For this review, take the finished solid that the model builds, in its own axes (mm). Face numbers are marked on the shaded views. A direction names the side the tool comes from. Give positions to 0.01 mm unless a question says otherwise; leave off trailing zeros. Write each loop counter-clockwise with the first axis right and the second up, starting at its lowest first coordinate (ties: lowest second). Pieces come first, ordered by that corner, then holes. Notation, with made-up numbers: M 73.5,54.5 L 95.5,54.5 A26 cw 95.5,86.5 Z; hole C 79.25,40 d2. An arc over 180 degrees is marked long. One line per item, written item: value. Start each with the question number.
Item 1: Consider section D-D, the plane z = 32.1. Write out the cut boundary in (x, y).
Item 2: Consider section C-C, the plane z = 14.9. Write out the cut boundary in (x, y), and give its area (3 significant figures).
Item 3: Consider section A-A, the plane x = -19.3. Write out the cut boundary in (y, z), and give its area (3 significant figures).
Item 4: Clearance check with flat-ended pins moving along their axes: pin 1 Ø16 at (x, z) = (-3.5, 25) entering from -Y; pin 2 Ø16 at (x, z) = (-7, 0.5) entering from -Y. State where each tip first meets the part, or that it passes through.
Item 5: Consider section B-B, the plane x = 0. Write out the cut boundary in (y, z).
Item 6: To check wall thickness, follow probe 1 along Z at (x, y) = (-34.4, -1.1); probe 2 along Z at (x, y) = (-20, -2.55); probe 3 along Z at (x, y) = (7.5, -4.6). State the ranges of each line that lie inside material, in increasing order.
Item 7: Tool access review of the marked faces 4 and 5: name each direction out of +Z, -Z, +X, -X, +Y, -Y from which nothing blocks a thin tool from reaching the whole face with its end or side.
Item 8: Mouldability with a two-part tool opening along X and no side actions: class the marked faces 1, 2 and 3 as released by +X, released by -X, zero draft, split by the parting line, or undercut.
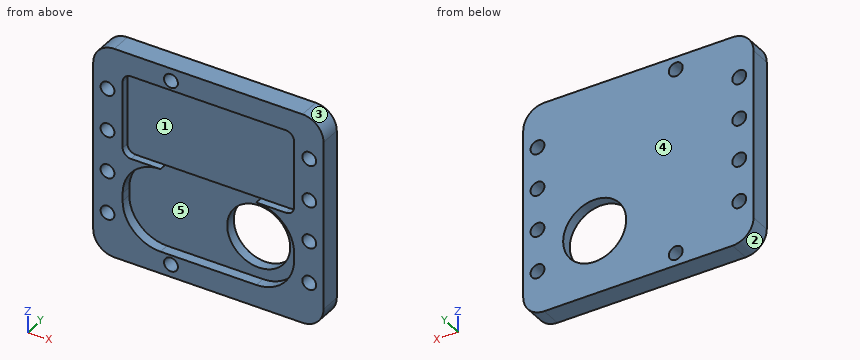
```python
from build123d import *

# Parameters (mm, degrees)
EXTRUSION1_DEPTH        = 5
ENL_V_MAT_EXTRU_2_DEPTH = 2.5
ENL_V_MAT_EXTRU_4_DEPTH = 1.8
ESQUISSE7_R             = 7.5
ENL_V_MAT_EXTRU_3_DEPTH = 52.643973511
TROU_TARAUD_M4X0_71_D   = 3.3


with BuildPart() as part:
    # Esquisse1 → Extrusion1 (new body)
    with BuildSketch(Plane(origin=(0, 0, 0), x_dir=(1, 0, 0), z_dir=(0, 1, 0))):
        with BuildLine():
            Line((-32.8, -35.1), (12, -35.1))
            ThreePointArc((12, -35.1), (15.535533906, -33.635533906), (17, -30.1))
            Line((17, -30.1), (17, 10.2))
            ThreePointArc((17, 10.2), (15.535533906, 13.735533906), (12, 15.2))
            Line((12, 15.2), (-32.8, 15.2))
            ThreePointArc((-32.8, 15.2), (-36.335533906, 13.735533906), (-37.8, 10.2))
            Line((-37.8, 10.2), (-37.8, -30.1))
            ThreePointArc((-37.8, -30.1), (-36.335533906, -33.635533906), (-32.8, -35.1))
        make_face()
    extrude(amount=-EXTRUSION1_DEPTH)

    # Esquisse6 → Enlèv. mat.-Extru.2 (cut)
    with BuildSketch(Plane.XZ.offset(5)):
        with BuildLine():
            Line((1, 9.95), (-21.8, 9.95))
            ThreePointArc((-21.8, 9.95), (-28.163961031, 7.313961031), (-30.8, 0.95))
            Line((-30.8, 0.95), (-30.8, -0.95))
            ThreePointArc((-30.8, -0.95), (-28.163961031, -7.313961031), (-21.8, -9.95))
            Line((-21.8, -9.95), (1, -9.95))
            ThreePointArc((1, -9.95), (7.363961031, -7.313961031), (10, -0.95))
            Line((10, -0.95), (10, 0.95))
            ThreePointArc((10, 0.95), (7.363961031, 7.313961031), (1, 9.95))
        make_face()
    extrude(amount=-ENL_V_MAT_EXTRU_2_DEPTH, mode=Mode.SUBTRACT)

    # Esquisse10 → Enlèv. mat.-Extru.4 (cut)
    with BuildSketch(Plane.XZ.offset(5)):
        with BuildLine():
            Line((8, 9.95), (-28.8, 9.95))
            ThreePointArc((-28.8, 9.95), (-30.214213562, 10.535786438), (-30.8, 11.95))
            Line((-30.8, 11.95), (-30.8, 27.85))
            ThreePointArc((-30.8, 27.85), (-30.214213562, 29.264213562), (-28.8, 29.85))
            Line((-28.8, 29.85), (8, 29.85))
            ThreePointArc((8, 29.85), (9.414213562, 29.264213562), (10, 27.85))
            Line((10, 27.85), (10, 11.95))
            ThreePointArc((10, 11.95), (9.414213562, 10.535786438), (8, 9.95))
        make_face()
    extrude(amount=-ENL_V_MAT_EXTRU_4_DEPTH, mode=Mode.SUBTRACT)

    # Esquisse7 → Enlèv. mat.-Extru.3 (cut, through all)
    with BuildSketch(Plane.XZ.offset(2.5)):
        Circle(ESQUISSE7_R)
    extrude(amount=-ENL_V_MAT_EXTRU_3_DEPTH, mode=Mode.SUBTRACT)

    # Trou taraudé M4x0.71 (through all)
    with Locations(Plane.XZ.offset(5)):
        with Locations((-34.4, 5), (-34.4, -5), (13.6, 5), (13.6, -5), (-19.3, -12.2), (-19.3, 32.1), (13.6, 24.9), (13.6, 14.9), (-34.4, 14.9), (-34.4, 24.9)):
            Hole(TROU_TARAUD_M4X0_71_D / 2)


solid = part.part
```
Model answer:
1. outline: M -37.38,-5 L -20.95,-5 L -20.95,0 L -37.38,0 Z; M -17.65,-5 L 16.58,-5 L 16.58,0 L -17.65,0 Z
2. outline: M -37.8,-5 L -36.05,-5 L -36.05,0 L -37.8,0 Z; M -32.75,-5 L -30.8,-5 L -30.8,-3.2 L 10,-3.2 L 10,-5 L 11.95,-5 L 11.95,0 L -32.75,0 Z; M 15.25,-5 L 17,-5 L 17,0 L 15.25,0 Z
2. area: 168 mm2
3. outline: M -5,-15.2 L 0,-15.2 L 0,-13.85 L -5,-13.85 Z; M -5,-10.55 L 0,-10.55 L 0,30.45 L -5,30.45 L -5,29.85 L -3.2,29.85 L -3.2,9.95 L -2.5,9.95 L -2.5,-9.95 L -5,-9.95 Z; M -5,33.75 L 0,33.75 L 0,35.1 L -5,35.1 Z
3. area: 133 mm2
4. pin 1: stops at y = -5
4. pin 2: stops at y = -2.5
5. outline: M -5,-15.2 L 0,-15.2 L 0,-7.5 L -2.5,-7.5 L -2.5,-9.95 L -5,-9.95 Z; M -5,29.85 L -3.2,29.85 L -3.2,9.95 L -2.5,9.95 L -2.5,7.5 L 0,7.5 L 0,35.1 L -5,35.1 Z
6. probe 1: z = -14.94 to -6.65, -3.35 to 3.35, 6.65 to 13.25, 16.55 to 23.25, 26.55 to 34.84
6. probe 2: z = -15.2 to -13.69, -10.71 to -9.95, 9.95 to 30.61, 33.59 to 35.1
6. probe 3: z = -15.2 to -7.17, 7.17 to 9.95, 29.85 to 35.1
7. face 4: +Z, -Z, +X, -X, +Y
7. face 5: -Y
8. face 1: undercut
8. face 2: released by -X
8. face 3: released by +X
